from build123d import *

# Parameters (mm, degrees)
SKETCH2_W              = 120
SKETCH2_H              = 15
BOSS_EXTRUDE1_DEPTH    = 150
BOSS_EXTRUDE3_DEPTH    = 150
SKETCH7_W              = 112
SKETCH7_H              = 140
CUT_EXTRUDE1_DEPTH     = 165.890873004
SKETCH8_W              = 92
SKETCH8_H              = 120
CUT_EXTRUDE2_DEPTH     = 165.890873004
SKETCH12_OUTSIDE_W     = 161.458
SKETCH12_OUTSIDE_H     = 191.458
SKETCH12_OUTSIDE_W_2   = 110
SKETCH12_OUTSIDE_H_2   = 140
CUT_EXTRUDE5_DEPTH     = 5
BOSS_EXTRUDE4_REACH    = 163.342
SKETCH14_W             = 112
SKETCH14_H             = 3
CUT_EXTRUDE6_REACH     = 165.495
SKETCH15_W             = 102
SKETCH15_H             = 130
SKETCH16_W             = 5
SKETCH16_H             = 6
BOSS_EXTRUDE5_DEPTH    = 6
CUT_EXTRUDE7_REACH     = 170.114
SKETCH17_W             = 3
SKETCH17_H             = 3
FILLET1_R              = 2
LPATTERN1_COUNT        = 5
LPATTERN1_PITCH        = 36.25
FILLET1_OF_LPATTERN1_R = 2
MIRROR1_DEPTH          = 5
MIRROR1_START          = 36.25
MIRROR1_2_DEPTH        = 5
MIRROR1_START_2        = 72.5
MIRROR1_3_DEPTH        = 5
MIRROR1_START_3        = 108.75
MIRROR1_4_DEPTH        = 5
MIRROR1_START_4        = 145
MIRROR1_5_DEPTH        = 5
SKETCH18_W             = 5
SKETCH18_H             = 6
BOSS_EXTRUDE6_DEPTH    = 6
CUT_EXTRUDE8_REACH     = 171.111
SKETCH19_W             = 3
SKETCH19_H             = 3
FILLET2_R              = 2
FILLET2_OF_MIRROR2_R   = 2
SKETCH20_R             = 23
CUT_EXTRUDE9_DEPTH     = 3
SKETCH21_W             = 18
SKETCH21_H             = 6
CUT_EXTRUDE10_DEPTH    = 2


# Read off the part's stored shape, not the designer's step: Mirror1
with BuildPart() as part:
    # Sketch2 → Boss-Extrude1 (new body)
    with BuildSketch(Plane.XY):
        Rectangle(SKETCH2_W, SKETCH2_H)
    extrude(amount=BOSS_EXTRUDE1_DEPTH)

    # Sketch4 → Boss-Extrude3 (add)
    with BuildSketch(Plane(origin=(0, 0, 0), x_dir=(-1, 0, 0), z_dir=(0, 0, -1))):
        with BuildLine():
            Line((-60, 7.5), (60, 7.5))
            ThreePointArc((60, 7.5), (0, 37.5), (-60, 7.5))
        make_face()
    extrude(amount=-BOSS_EXTRUDE3_DEPTH)

    # Sketch7 → Cut-Extrude1 (cut, through all)
    with BuildSketch(Plane(origin=(0, 4.5, 0), x_dir=(-1, 0, 0), z_dir=(0, -1, 0))):
        with Locations((0, -75)):
            Rectangle(SKETCH7_W, SKETCH7_H)
    extrude(amount=-CUT_EXTRUDE1_DEPTH, mode=Mode.SUBTRACT)

    # Sketch8 → Cut-Extrude2 (cut, through all)
    with BuildSketch(Plane(origin=(0, 4.5, 0), x_dir=(1, 0, 0), z_dir=(0, 1, 0))):
        with Locations((0, -75)):
            Rectangle(SKETCH8_W, SKETCH8_H)
    extrude(amount=-CUT_EXTRUDE2_DEPTH, mode=Mode.SUBTRACT)

    # Sketch12 outside → Cut-Extrude5 (cut)
    with BuildSketch(Plane(origin=(0, -7.5, 0), x_dir=(-1, 0, 0), z_dir=(0, -1, 0))):
        with Locations((0, -75)):
            Rectangle(SKETCH12_OUTSIDE_W, SKETCH12_OUTSIDE_H)
        with Locations((0, -75)):
            Rectangle(SKETCH12_OUTSIDE_W_2, SKETCH12_OUTSIDE_H_2, mode=Mode.SUBTRACT)
    extrude(amount=-CUT_EXTRUDE5_DEPTH, mode=Mode.SUBTRACT)

    # Sketch14 → Boss-Extrude4 (add, up to next)
    with BuildSketch(Plane.XY.offset(5), mode=Mode.PRIVATE) as boss_extrude4_sk1:
        with Locations((0, 10.889878733)):
            Rectangle(SKETCH14_W, SKETCH14_H)
    boss_extrude4_tool1 = extrude(boss_extrude4_sk1.sketch, amount=BOSS_EXTRUDE4_REACH, mode=Mode.PRIVATE) - part.part
    add(boss_extrude4_tool1.solids().sort_by_distance((0, 10.889879, 5))[0])

    # Sketch15 → Cut-Extrude6 (cut, up to next)
    with BuildSketch(Plane(origin=(0, 12.389878733, 0), x_dir=(1, 0, 0), z_dir=(0, 1, 0)), mode=Mode.PRIVATE) as cut_extrude6_sk1:
        with Locations((0, -75)):
            Rectangle(SKETCH15_W, SKETCH15_H)
    cut_extrude6_tool1 = extrude(cut_extrude6_sk1.sketch, amount=-CUT_EXTRUDE6_REACH, mode=Mode.PRIVATE) & part.part
    add(cut_extrude6_tool1.solids().sort_by_distance((0, 12.389879, 75))[0], mode=Mode.SUBTRACT)

    # Sketch16 → Boss-Extrude5 (add)
    with BuildSketch(Plane(origin=(60, 0, 0), x_dir=(0, 0, -1), z_dir=(1, 0, 0))):
        with Locations((-2.5, 0.5)):
            Rectangle(SKETCH16_W, SKETCH16_H)
    boss_extrude5 = extrude(amount=BOSS_EXTRUDE5_DEPTH)

    # Sketch17 → Cut-Extrude7 (cut, up to next)
    with BuildSketch(Plane(origin=(0, 0, 0), x_dir=(-1, 0, 0), z_dir=(0, 0, -1)), mode=Mode.PRIVATE) as cut_extrude7_sk1:
        with Locations((-61.5, 2)):
            Rectangle(SKETCH17_W, SKETCH17_H)
    cut_extrude7_tool1 = extrude(cut_extrude7_sk1.sketch, amount=-CUT_EXTRUDE7_REACH, mode=Mode.PRIVATE) & part.part
    cut_extrude7 = cut_extrude7_tool1.solids().sort_by_distance((61.5, 2, 0))[0]
    add(cut_extrude7, mode=Mode.SUBTRACT)

    # Fillet1
    fillet1_edges = [part.edges().sort_by_distance(p)[0] for p in [
        (66, 3.5, 2.5),
        (66, -2.5, 2.5),
    ]]
    fillet(fillet1_edges, radius=FILLET1_R)

    # LPattern1: Boss-Extrude5, Cut-Extrude7 ×5
    with Locations(*[(0, 0, i * LPATTERN1_PITCH) for i in range(1, LPATTERN1_COUNT)]):
        add(boss_extrude5)
        add(cut_extrude7, mode=Mode.SUBTRACT)

    # Fillet1 of LPattern1
    fillet1_of_lpattern1_edges = [part.edges().sort_by_distance(p)[0] for p in [
        (66, 3.5, 38.75),
        (66, -2.5, 38.75),
        (66, 3.5, 75),
        (66, -2.5, 75),
        (66, 3.5, 111.25),
        (66, -2.5, 111.25),
        (66, 3.5, 147.5),
        (66, -2.5, 147.5),
    ]]
    fillet(fillet1_of_lpattern1_edges, radius=FILLET1_OF_LPATTERN1_R)

    # Mirror1 outline → Mirror1 (add)
    with BuildSketch(Plane.XY):
        with BuildLine():
            Line((-63, 0.5), (-63, 3.5))
            Line((-63, 3.5), (-64, 3.5))
            ThreePointArc((-64, 3.5), (-65.414213562, 2.914213562), (-66, 1.5))
            Line((-66, 1.5), (-66, -0.5))
            ThreePointArc((-66, -0.5), (-65.414213562, -1.914213562), (-64, -2.5))
            Line((-64, -2.5), (-60, -2.5))
            Line((-60, -2.5), (-60, 0.5))
            Line((-60, 0.5), (-63, 0.5))
        make_face()
    extrude(amount=MIRROR1_DEPTH)

    # Mirror1 2 outline → Mirror1 2 (add)
    with BuildSketch(Plane.XY.offset(MIRROR1_START)):
        with BuildLine():
            Line((-63, 0.5), (-63, 3.5))
            Line((-63, 3.5), (-64, 3.5))
            ThreePointArc((-64, 3.5), (-65.414213562, 2.914213562), (-66, 1.5))
            Line((-66, 1.5), (-66, -0.5))
            ThreePointArc((-66, -0.5), (-65.414213562, -1.914213562), (-64, -2.5))
            Line((-64, -2.5), (-60, -2.5))
            Line((-60, -2.5), (-60, 0.5))
            Line((-60, 0.5), (-63, 0.5))
        make_face()
    extrude(amount=MIRROR1_2_DEPTH)

    # Mirror1 3 outline → Mirror1 3 (add)
    with BuildSketch(Plane.XY.offset(MIRROR1_START_2)):
        with BuildLine():
            Line((-63, 0.5), (-63, 3.5))
            Line((-63, 3.5), (-64, 3.5))
            ThreePointArc((-64, 3.5), (-65.414213562, 2.914213562), (-66, 1.5))
            Line((-66, 1.5), (-66, -0.5))
            ThreePointArc((-66, -0.5), (-65.414213562, -1.914213562), (-64, -2.5))
            Line((-64, -2.5), (-60, -2.5))
            Line((-60, -2.5), (-60, 0.5))
            Line((-60, 0.5), (-63, 0.5))
        make_face()
    extrude(amount=MIRROR1_3_DEPTH)

    # Mirror1 4 outline → Mirror1 4 (add)
    with BuildSketch(Plane.XY.offset(MIRROR1_START_3)):
        with BuildLine():
            Line((-63, 0.5), (-63, 3.5))
            Line((-63, 3.5), (-64, 3.5))
            ThreePointArc((-64, 3.5), (-65.414213562, 2.914213562), (-66, 1.5))
            Line((-66, 1.5), (-66, -0.5))
            ThreePointArc((-66, -0.5), (-65.414213562, -1.914213562), (-64, -2.5))
            Line((-64, -2.5), (-60, -2.5))
            Line((-60, -2.5), (-60, 0.5))
            Line((-60, 0.5), (-63, 0.5))
        make_face()
    extrude(amount=MIRROR1_4_DEPTH)

    # Mirror1 5 outline → Mirror1 5 (add)
    with BuildSketch(Plane.XY.offset(MIRROR1_START_4)):
        with BuildLine():
            Line((-63, 0.5), (-63, 3.5))
            Line((-63, 3.5), (-64, 3.5))
            ThreePointArc((-64, 3.5), (-65.414213562, 2.914213562), (-66, 1.5))
            Line((-66, 1.5), (-66, -0.5))
            ThreePointArc((-66, -0.5), (-65.414213562, -1.914213562), (-64, -2.5))
            Line((-64, -2.5), (-60, -2.5))
            Line((-60, -2.5), (-60, 0.5))
            Line((-60, 0.5), (-63, 0.5))
        make_face()
    extrude(amount=MIRROR1_5_DEPTH)

    # Sketch18 → Boss-Extrude6 (add)
    with BuildSketch(Plane(origin=(0, 0, 0), x_dir=(-1, 0, 0), z_dir=(0, 0, -1))):
        with Locations((0, 0.5)):
            Rectangle(SKETCH18_W, SKETCH18_H)
    boss_extrude6 = extrude(amount=BOSS_EXTRUDE6_DEPTH)

    # Sketch19 → Cut-Extrude8 (cut, up to next)
    with BuildSketch(Plane(origin=(2.5, 0, 0), x_dir=(0, 0, -1), z_dir=(1, 0, 0)), mode=Mode.PRIVATE) as cut_extrude8_sk1:
        with Locations((1.5, 2)):
            Rectangle(SKETCH19_W, SKETCH19_H)
    cut_extrude8_tool1 = extrude(cut_extrude8_sk1.sketch, amount=-CUT_EXTRUDE8_REACH, mode=Mode.PRIVATE) & part.part
    cut_extrude8 = cut_extrude8_tool1.solids().sort_by_distance((2.5, 2, -1.5))[0]
    add(cut_extrude8, mode=Mode.SUBTRACT)

    # Fillet2
    fillet2_edges = [part.edges().sort_by_distance(p)[0] for p in [
        (0, -2.5, -6),
        (0, 3.5, -6),
    ]]
    fillet(fillet2_edges, radius=FILLET2_R)

    # Mirror2: Boss-Extrude6, Cut-Extrude8 across plane
    add(boss_extrude6.mirror(Plane.XY.offset(75)))
    add(cut_extrude8.mirror(Plane.XY.offset(75)), mode=Mode.SUBTRACT)

    # Fillet2 of Mirror2
    fillet2_of_mirror2_edges = [part.edges().sort_by_distance(p)[0] for p in [
        (0, -2.5, 156),
        (0, 3.5, 156),
    ]]
    fillet(fillet2_of_mirror2_edges, radius=FILLET2_OF_MIRROR2_R)

    # Sketch20 → Cut-Extrude9 (cut)
    with BuildSketch(Plane(origin=(0, -7.5, 0), x_dir=(-1, 0, 0), z_dir=(0, -1, 0))):
        with Locations((30, -102.5)):
            Circle(SKETCH20_R)
        with Locations((-30, -47.5)):
            Circle(SKETCH20_R)
    extrude(amount=-CUT_EXTRUDE9_DEPTH, mode=Mode.SUBTRACT)

    # Sketch21 → Cut-Extrude10 (cut)
    with BuildSketch(Plane(origin=(0, -7.5, 0), x_dir=(-1, 0, 0), z_dir=(0, -1, 0))):
        with Locations((0, -138)):
            Rectangle(SKETCH21_W, SKETCH21_H)
    cut_extrude10 = extrude(amount=-CUT_EXTRUDE10_DEPTH, mode=Mode.SUBTRACT)

    # Mirror3: Cut-Extrude10 across plane
    add(cut_extrude10.mirror(Plane.XY.offset(75)), mode=Mode.SUBTRACT)


solid = part.part
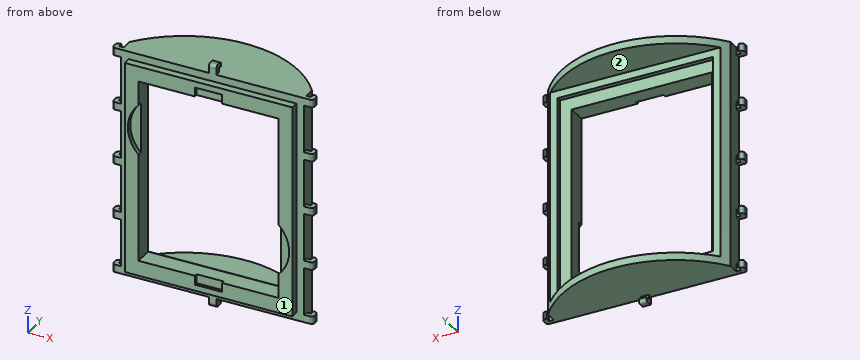
The listing builds one solid part. Answer for the finished solid, in the listing's coordinates (mm). Face numbers are marked on the shaded views. Give positions to 0.01 mm unless a question says otherwise; leave off trailing zeros. Loops run counter-clockwise (first coordinate to the right, second up) from the corner with the lowest first, then second, coordinate; pieces in that order, holes last.
Item 1: A cutting plane is placed at D-D (x = 26.5). Give the vertices of the cut face in (y, z), then the cut area to 3 significant figures.
Derived:
outline: (-7.5, 5) - (-2.5, 5) - (-2.5, 0) - (32.66, 0) - (32.66, 5) - (12.39, 5) - (12.39, 10) - (9.39, 10) - (9.39, 5) - (4.5, 5) - (4.5, 15) - (-7.5, 15) - close; (-7.5, 135) - (4.5, 135) - (4.5, 145) - (9.39, 145) - (9.39, 140) - (12.39, 140) - (12.39, 145) - (32.66, 145) - (32.66, 150) - (-2.5, 150) - (-2.5, 145) - (-7.5, 145) - close
area: 622 mm2
Item 2: Determine the mould class of the marked faces 1 and 2 for opening direction Z: +Z half, -Z half, draft (parallel to the pull), parting line (faces both ways), or undercut.
Derived:
face 1: draft
face 2: undercut
Item 3: A cutting plane is placed at A-A (x = -21). Give the vertices of the cut face in (y, z).
Derived:
outline: (-7.5, 5) - (-2.5, 5) - (-2.5, 0) - (34.5, 0) - (34.5, 5) - (12.39, 5) - (12.39, 10) - (9.39, 10) - (9.39, 5) - (4.5, 5) - (4.5, 15) - (-7.5, 15) - close; (-7.5, 135) - (4.5, 135) - (4.5, 145) - (9.39, 145) - (9.39, 140) - (12.39, 140) - (12.39, 145) - (34.5, 145) - (34.5, 150) - (-2.5, 150) - (-2.5, 145) - (-7.5, 145) - close
Item 4: Each of these flat-tipped pins is pushed along its axis until it touches: pin 1 Ø3.5 at (x, y) = (5, 11.5) entering from -Z; pin 2 Ø8 at (x, y) = (-40, 1) entering from +Z; pin 3 Ø6 at (y, z) = (-3, 85.5) entering from +X. Where does it stop, or does it pass through?
Derived:
pin 1: stops at z = 0
pin 2: stops at z = 150
pin 3: stops at x = 60
Item 5: A cutting plane is placed at C-C (y = 20.5). Give the vertices of the cut face in (x, z).
Derived:
outline: (-47.55, 0) - (47.55, 0) - (47.55, 5) - (-47.55, 5) - close; (-47.55, 145) - (47.55, 145) - (47.55, 150) - (-47.55, 150) - close
Item 6: A cutting plane is placed at B-B (z = 131). Give the vertices of the cut face in (x, y).
Derived:
outline: (-60, -2.5) - (-55, -2.5) - (-55, -7.5) - (-46, -7.5) - (-46, 4.5) - (-56, 4.5) - (-56, 9.39) - (-51, 9.39) - (-51, 12.39) - (-56, 12.39) arc R75 ccw to (-60, 7.5) - close; (46, -7.5) - (55, -7.5) - (55, -2.5) - (60, -2.5) - (60, 7.5) arc R75 ccw to (56, 12.39) - (51, 12.39) - (51, 9.39) - (56, 9.39) - (56, 4.5) - (46, 4.5) - close
Item 7: Find the intervals of material crossed by line 1 along Z through (x, y) = (22, 34); line 2 along X through (y, z) = (-3, 42.5); line 3 along Z through (x, y) = (2.5, 4), in increasing order.
Derived:
line 1: z = 0 to 5, 145 to 150
line 2: x = -55 to -46, 46 to 55
line 3: z = 0 to 15, 135 to 150
